Verification items for the finished model (mm, model axes). Face numbers are marked on the shaded views. Coordinates: 2 decimals unless noted, no trailing zeros. Order: outer loops, then holes, each group sorted by start corner. A loop starts at its lowest first (then second) coordinate and runs counter-clockwise, first axis right, second up. Notation, with made-up numbers: M 12,55.25 L 43,55.25 A22 ccw 43,71.25 Z; hole C 32.5,17 d4. An arc over 180 degrees is marked long. Return JSON: item names as keys, results as strings.
```python
from build123d import *

# Parameters (mm, degrees)
F0_R     = 74.1026
F1_DEPTH = 12.7
F2_DEPTH = 6.35
F3_DEPTH = 12.7
F4_R     = 1.905


with BuildPart() as f1:
    # F0 (on Front) → F1 (new body, symmetric)
    with BuildSketch(Plane.XZ):
        Circle(F0_R)
        with BuildLine():
            Line((12.7, -56.305081), (12.7, 56.305081))
            ThreePointArc((12.7, 56.305081), (45.16875, 36.037206), (58.065501, 0))
            ThreePointArc((58.065501, 0), (45.258761, -36.10973), (12.7, -56.305081))
        make_face(mode=Mode.SUBTRACT)
        with BuildLine():
            ThreePointArc((-58.065501, 0), (-45.16875, 36.037206), (-12.7, 56.305081))
            Line((-12.7, 56.305081), (-12.7, -56.305081))
            ThreePointArc((-12.7, -56.305081), (-46.002553, -36.709009), (-58.065501, 0))
        make_face(mode=Mode.SUBTRACT)
    extrude(amount=F1_DEPTH, both=True)

    # F0 (on Front) → F2 (join, symmetric)
    with BuildSketch(Plane.XZ):
        with BuildLine():
            Line((-12.7, -56.305081), (-12.7, 56.305081))
            ThreePointArc((-12.7, 56.305081), (-45.16875, 36.037206), (-58.065501, 0))
            ThreePointArc((-58.065501, 0), (-46.002553, -36.709009), (-12.7, -56.305081))
        make_face()
        with BuildLine():
            Line((-43.460501, 0), (-20.32, -10.472688))
            ThreePointArc((-20.32, -10.472688), (-21.550138, -12.848968), (-23.023436, -15.082651))
            ThreePointArc((-23.023436, -15.082651), (-28.261599, -17.66068), (-33.390806, -14.872163))
            Line((-33.390806, -14.872163), (-43.460501, 0))
        make_face(mode=Mode.SUBTRACT)
        with BuildLine():
            ThreePointArc((58.065501, 0), (45.16875, 36.037206), (12.7, 56.305081))
            Line((12.7, 56.305081), (12.7, -56.305081))
            ThreePointArc((12.7, -56.305081), (45.258761, -36.10973), (58.065501, 0))
        make_face()
        with BuildLine():
            ThreePointArc((22.929982, -14.532426), (21.511965, -12.57522), (20.32, -10.472688))
            Line((20.32, -10.472688), (43.460501, 0))
            Line((43.460501, 0), (32.976203, -14.284045))
            ThreePointArc((32.976203, -14.284045), (28.014074, -16.874772), (22.929982, -14.532426))
        make_face(mode=Mode.SUBTRACT)
    extrude(amount=F2_DEPTH, both=True)

    # F0 (on Front) → F3 (join, symmetric)
    with BuildSketch(Plane.XZ):
        with BuildLine():
            ThreePointArc((-23.023436, -15.082651), (-21.550138, -12.848968), (-20.32, -10.472688))
            Line((-20.32, -10.472688), (-43.460501, 0))
            Line((-43.460501, 0), (-33.390806, -14.872163))
            ThreePointArc((-33.390806, -14.872163), (-28.261599, -17.66068), (-23.023436, -15.082651))
        make_face()
        with BuildLine():
            Line((43.460501, 0), (20.32, -10.472688))
            ThreePointArc((20.32, -10.472688), (21.511965, -12.57522), (22.929982, -14.532426))
            ThreePointArc((22.929982, -14.532426), (28.014074, -16.874772), (32.976203, -14.284045))
            Line((32.976203, -14.284045), (43.460501, 0))
        make_face()
    extrude(amount=F3_DEPTH, both=True)

    # F4
    f4_edges = [f1.edges().sort_by_distance(p)[0] for p in [
        (-38.425654, -12.7, -7.436082),
        (38.218352, -12.7, -7.142023),
        (-31.890251, -12.7, -5.236344),
        (31.890251, -12.7, -5.236344),
    ]]
    fillet(f4_edges, radius=F4_R)


solid = f1.part
```
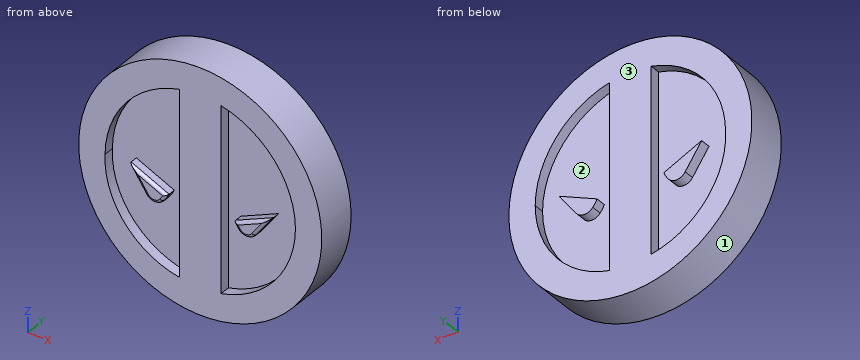
Q1. Cross-section at B-B, the plane x = -49. Record the boundary of the cut face in (y, z).
Values:
{"outline": "M -12.7,-55.59 L 12.7,-55.59 L 12.7,-32.61 L 6.35,-32.61 L 6.35,30.69 L 12.7,30.69 L 12.7,55.59 L -12.7,55.59 L -12.7,30.69 L -6.35,30.69 L -6.35,-32.61 L -12.7,-32.61 Z"}
Q2. Go/stop test with flat-tipped pins: pin 1 (7 mm diameter, centred on y = -8.5, z = 10.5, fed in from -X); pin 2 (5 mm diameter, centred on y = -9.5, z = -13.5, fed in from +X); pin 3 (10 mm diameter, centred on x = 44.5, y = 0, fed in from -Z). Record where each tip stops, or that it passes through.
Values:
{"pin 1": "x = -73.77", "pin 2": "x = 73.28", "pin 3": "z = -62.7"}
Q3. Draft check along Z on the marked faces 1, 2 and 3. Enter one of: pulls with the +Z half, pulls with the -Z half, needs draft (parallel to the pull), parting line crosses it, or undercut.
Values:
{"face 1": "parting line crosses it", "face 2": "undercut", "face 3": "needs draft"}
Q4. Cross-section at A-A, the plane y = 10.75. Record the boundary of the cut face in (x, z), and give its area (3 significant figures).
Values:
{"outline": "C 0,0 d148.21; M -43.46,0 L -33.39,-14.87 A6.35 ccw -23.02,-15.08 A25.4 ccw -20.32,-10.47 Z; M 20.32,-10.47 A21.74 ccw 22.93,-14.53 A6.35 ccw 32.98,-14.28 L 43.46,0 Z; hole M -58.07,0 A54.74 ccw -12.7,-56.31 L -12.7,56.31 A58.29 ccw Z; hole M 12.7,-56.31 A57.87 ccw 58.07,0 A58.29 ccw 12.7,56.31 Z", "area": "9,910 mm^2"}
Q5. Material ranges on line 1 along X through (y, z) = (-11, 1.5); line 2 along X through (y, z) = (-8.75, -31); line 3 along Z through (x, y) = (40, 8.5), recorded low to high.
Values:
{"line 1": "-74.09 to -58.03, -12.7 to 12.7, 58.03 to 74.09", "line 2": "-67.31 to -50.03, -12.7 to 12.7, 48.94 to 67.31", "line 3": "-62.38 to -41.81, -4.71 to -1.57, 41.66 to 62.38"}
Q6. Cross-section at D-D, the plane y = -3.25. Record the boundary of the cut face in (x, z), and give its area (3 significant figures).
Values:
{"outline": "C 0,0 d148.21", "area": "17,300 mm^2"}
Q7. Cross-section at C-C, the plane z = -40.5. Record the boundary of the cut face in (x, y), and give its area (3 significant figures).
Values:
{"outline": "M -62.06,-12.7 L -42.65,-12.7 L -42.65,-6.35 L -12.7,-6.35 L -12.7,-12.7 L 12.7,-12.7 L 12.7,-6.35 L 41.34,-6.35 L 41.34,-12.7 L 62.06,-12.7 L 62.06,12.7 L 41.34,12.7 L 41.34,6.35 L 12.7,6.35 L 12.7,12.7 L -12.7,12.7 L -12.7,6.35 L -42.65,6.35 L -42.65,12.7 L -62.06,12.7 Z", "area": "2,410 mm^2"}
